Source: CAD feature listing. Evaluate the final solid. Frame: model axes, mm. A direction names the side the tool comes from. Give positions to 0.01 mm unless a question says otherwise; leave off trailing zeros. Loops run counter-clockwise (first coordinate to the right, second up) from the corner with the lowest first, then second, coordinate; pieces in that order, holes last. Notation, with made-up numbers: M 24.25,-31 L 44.25,-31 A27 ccw 44.25,-2 Z; hole C 18.5,-23 d2. An arc over 180 degrees is marked long. Answer in a Markdown table with one row per item.
```python
from build123d import *

# Parameters (mm, degrees)
BOSS_EXTRUDE1_DEPTH         = 2
SKETCH5_R                   = 4.5
SKETCH5_R_2                 = 2.5
BOSS_EXTRUDE2_DEPTH         = 3
SKETCH8_R                   = 1.5
CUT_EXTRUDE2_DEPTH          = 28.531284582
CUT_EXTRUDE3_REACH          = 29.531
SKETCH10_R                  = 0.75
LPATTERN1_COUNT             = 4
LPATTERN1_PITCH             = 3
CIRPATTERN1_COUNT           = 4
CIRPATTERN1_COPY_1_REACH    = 29.531
CIRPATTERN1_COPY_1_SKETCH_R = 0.75
CIRPATTERN1_COPY_2_REACH    = 29.531
CIRPATTERN1_COPY_2_SKETCH_R = 0.75
CIRPATTERN1_COPY_3_REACH    = 29.531
CIRPATTERN1_COPY_3_SKETCH_R = 0.75
CIRPATTERN1_COPY_4_REACH    = 29.531
CIRPATTERN1_COPY_4_SKETCH_R = 0.75
CIRPATTERN1_COPY_5_REACH    = 29.531
CIRPATTERN1_COPY_5_SKETCH_R = 0.75
CIRPATTERN1_COPY_6_REACH    = 29.531
CIRPATTERN1_COPY_6_SKETCH_R = 0.75
CIRPATTERN1_COPY_7_REACH    = 29.531
CIRPATTERN1_COPY_7_SKETCH_R = 0.75
CIRPATTERN1_COPY_8_REACH    = 29.531
CIRPATTERN1_COPY_8_SKETCH_R = 0.75
CIRPATTERN1_COPY_9_REACH    = 29.531
CIRPATTERN1_COPY_9_SKETCH_R = 0.75
SKETCH9_R                   = 4.5
SKETCH9_R_2                 = 3.3
SKETCH9_R_3                 = 2.8
SKETCH9_R_4                 = 1.5
CUT_EXTRUDE4_DEPTH          = 1


with BuildPart() as part:
    # Sketch1 → Boss-Extrude1 (new body)
    with BuildSketch(Plane(origin=(0, 0, 0), x_dir=(1, 0, 0), z_dir=(0, 1, 0))):
        with BuildLine():
            Line((10.343686836, 2.276584719), (4.865650492, -6.089484718))
            ThreePointArc((4.865650492, -6.089484718), (3.897502175, -8.118293207), (4.865650492, -10.147101696))
            Line((4.865650492, -10.147101696), (10.343686836, -18.513171133))
            ThreePointArc((10.343686836, -18.513171133), (10.084686511, -21.022991964), (7.57486568, -21.281992289))
            Line((7.57486568, -21.281992289), (-0.791203757, -15.803955945))
            ThreePointArc((-0.791203757, -15.803955945), (-2.820012246, -14.835807628), (-4.848820735, -15.803955945))
            Line((-4.848820735, -15.803955945), (-13.214890172, -21.281992289))
            ThreePointArc((-13.214890172, -21.281992289), (-15.724711003, -21.022991964), (-15.983711328, -18.513171133))
            Line((-15.983711328, -18.513171133), (-10.505674984, -10.147101696))
            ThreePointArc((-10.505674984, -10.147101696), (-9.537526667, -8.118293207), (-10.505674984, -6.089484718))
            Line((-10.505674984, -6.089484718), (-15.983711328, 2.276584719))
            ThreePointArc((-15.983711328, 2.276584719), (-15.724711003, 4.78640555), (-13.214890172, 5.045405875))
            Line((-13.214890172, 5.045405875), (-4.848820735, -0.432630469))
            ThreePointArc((-4.848820735, -0.432630469), (-2.820012246, -1.400778786), (-0.791203757, -0.432630469))
            Line((-0.791203757, -0.432630469), (7.57486568, 5.045405875))
            ThreePointArc((7.57486568, 5.045405875), (10.084686511, 4.78640555), (10.343686836, 2.276584719))
        make_face()
    extrude(amount=BOSS_EXTRUDE1_DEPTH)

    # Sketch5 → Boss-Extrude2 (add)
    with BuildSketch(Plane(origin=(0, 2, 0), x_dir=(1, 0, 0), z_dir=(0, 1, 0))):
        with Locations(Location((-2.820012246, -8.118293207, 0), (0, 0, 90))):
            Circle(SKETCH5_R)
        with Locations(Location((-2.820012246, -8.118293207, 0), (0, 0, 270))):
            Circle(SKETCH5_R_2, mode=Mode.SUBTRACT)
    extrude(amount=BOSS_EXTRUDE2_DEPTH)

    # Sketch8 → Cut-Extrude2 (cut, through all)
    with BuildSketch(Plane.XZ):
        with Locations(Location((-2.820012246, 8.118293207, 0), (0, 0, 270))):
            Circle(SKETCH8_R)
    extrude(amount=-CUT_EXTRUDE2_DEPTH, mode=Mode.SUBTRACT)

    # Sketch10 → Cut-Extrude3 (cut, up to next)
    with BuildSketch(Plane.XZ, mode=Mode.PRIVATE) as cut_extrude3_sk1:
        with Locations(Location((8.670472948, -3.372191987, 0), (0, 0, 270))):
            Circle(SKETCH10_R)
    cut_extrude3_tool1 = extrude(cut_extrude3_sk1.sketch, amount=-CUT_EXTRUDE3_REACH, mode=Mode.PRIVATE) & part.part
    cut_extrude3 = cut_extrude3_tool1.solids().sort_by_distance((8.670473, 0, -3.372192))[0]
    add(cut_extrude3, mode=Mode.SUBTRACT)

    # LPattern1: Cut-Extrude3 ×4
    with Locations(*[Vector(-0.7071067811865462, 0, 0.7071067811865489) * (i * LPATTERN1_PITCH) for i in range(1, LPATTERN1_COUNT)]):
        add(cut_extrude3, mode=Mode.SUBTRACT)

    # CirPattern1: Cut-Extrude3 ×4 about axis
    cirpattern1_axis = Axis((-2.820012246, 0, 8.118293207), (0, 1, 0))
    for i in range(1, CIRPATTERN1_COUNT):
        add(cut_extrude3.rotate(cirpattern1_axis, i * 360 / CIRPATTERN1_COUNT), mode=Mode.SUBTRACT)

    # CirPattern1 copy 1 sketch → CirPattern1 copy 1 (cut, up to next)
    with BuildSketch(Plane(origin=(-8.81698511, 0, 7.419601305), x_dir=(0, 0, -1), z_dir=(0, -1, 0)), mode=Mode.PRIVATE) as cirpattern1_copy_1_sk1:
        with Locations(Location((8.670472948, -3.372191987, 0), (0, 0, 270))):
            Circle(CIRPATTERN1_COPY_1_SKETCH_R)
    cirpattern1_copy_1_tool1 = extrude(cirpattern1_copy_1_sk1.sketch, amount=-CIRPATTERN1_COPY_1_REACH, mode=Mode.PRIVATE) & part.part
    add(cirpattern1_copy_1_tool1.solids().sort_by_distance((-12.18917711, 0, -1.250871695))[0], mode=Mode.SUBTRACT)

    # CirPattern1 copy 2 sketch → CirPattern1 copy 2 (cut, up to next)
    with BuildSketch(Plane(origin=(-3.518704148, 0, 14.115266071), x_dir=(-1, 0, 0), z_dir=(0, -1, 0)), mode=Mode.PRIVATE) as cirpattern1_copy_2_sk1:
        with Locations(Location((8.670472948, -3.372191987, 0), (0, 0, 270))):
            Circle(CIRPATTERN1_COPY_2_SKETCH_R)
    cirpattern1_copy_2_tool1 = extrude(cirpattern1_copy_2_sk1.sketch, amount=-CIRPATTERN1_COPY_2_REACH, mode=Mode.PRIVATE) & part.part
    add(cirpattern1_copy_2_tool1.solids().sort_by_distance((-12.189177148, 0, 17.487458071))[0], mode=Mode.SUBTRACT)

    # CirPattern1 copy 3 sketch → CirPattern1 copy 3 (cut, up to next)
    with BuildSketch(Plane(origin=(3.176960618, 0, 8.81698511), x_dir=(0, 0, 1), z_dir=(0, -1, 0)), mode=Mode.PRIVATE) as cirpattern1_copy_3_sk1:
        with Locations(Location((8.670472948, -3.372191987, 0), (0, 0, 270))):
            Circle(CIRPATTERN1_COPY_3_SKETCH_R)
    cirpattern1_copy_3_tool1 = extrude(cirpattern1_copy_3_sk1.sketch, amount=-CIRPATTERN1_COPY_3_REACH, mode=Mode.PRIVATE) & part.part
    add(cirpattern1_copy_3_tool1.solids().sort_by_distance((6.549152618, 0, 17.48745811))[0], mode=Mode.SUBTRACT)

    # CirPattern1 copy 4 sketch → CirPattern1 copy 4 (cut, up to next)
    with BuildSketch(Plane(origin=(-6.695664766, 0, 9.540921648), x_dir=(0, 0, -1), z_dir=(0, -1, 0)), mode=Mode.PRIVATE) as cirpattern1_copy_4_sk1:
        with Locations(Location((8.670472948, -3.372191987, 0), (0, 0, 270))):
            Circle(CIRPATTERN1_COPY_4_SKETCH_R)
    cirpattern1_copy_4_tool1 = extrude(cirpattern1_copy_4_sk1.sketch, amount=-CIRPATTERN1_COPY_4_REACH, mode=Mode.PRIVATE) & part.part
    add(cirpattern1_copy_4_tool1.solids().sort_by_distance((-10.067856766, 0, 0.870448648))[0], mode=Mode.SUBTRACT)

    # CirPattern1 copy 5 sketch → CirPattern1 copy 5 (cut, up to next)
    with BuildSketch(Plane(origin=(-1.397383805, 0, 11.993945727), x_dir=(-1, 0, 0), z_dir=(0, -1, 0)), mode=Mode.PRIVATE) as cirpattern1_copy_5_sk1:
        with Locations(Location((8.670472948, -3.372191987, 0), (0, 0, 270))):
            Circle(CIRPATTERN1_COPY_5_SKETCH_R)
    cirpattern1_copy_5_tool1 = extrude(cirpattern1_copy_5_sk1.sketch, amount=-CIRPATTERN1_COPY_5_REACH, mode=Mode.PRIVATE) & part.part
    add(cirpattern1_copy_5_tool1.solids().sort_by_distance((-10.067856805, 0, 15.366137727))[0], mode=Mode.SUBTRACT)

    # CirPattern1 copy 6 sketch → CirPattern1 copy 6 (cut, up to next)
    with BuildSketch(Plane(origin=(1.055640274, 0, 6.695664766), x_dir=(0, 0, 1), z_dir=(0, -1, 0)), mode=Mode.PRIVATE) as cirpattern1_copy_6_sk1:
        with Locations(Location((8.670472948, -3.372191987, 0), (0, 0, 270))):
            Circle(CIRPATTERN1_COPY_6_SKETCH_R)
    cirpattern1_copy_6_tool1 = extrude(cirpattern1_copy_6_sk1.sketch, amount=-CIRPATTERN1_COPY_6_REACH, mode=Mode.PRIVATE) & part.part
    add(cirpattern1_copy_6_tool1.solids().sort_by_distance((4.427832274, 0, 15.366137766))[0], mode=Mode.SUBTRACT)

    # CirPattern1 copy 7 sketch → CirPattern1 copy 7 (cut, up to next)
    with BuildSketch(Plane(origin=(-4.574344422, 0, 11.662241992), x_dir=(0, 0, -1), z_dir=(0, -1, 0)), mode=Mode.PRIVATE) as cirpattern1_copy_7_sk1:
        with Locations(Location((8.670472948, -3.372191987, 0), (0, 0, 270))):
            Circle(CIRPATTERN1_COPY_7_SKETCH_R)
    cirpattern1_copy_7_tool1 = extrude(cirpattern1_copy_7_sk1.sketch, amount=-CIRPATTERN1_COPY_7_REACH, mode=Mode.PRIVATE) & part.part
    add(cirpattern1_copy_7_tool1.solids().sort_by_distance((-7.946536422, 0, 2.991768992))[0], mode=Mode.SUBTRACT)

    # CirPattern1 copy 8 sketch → CirPattern1 copy 8 (cut, up to next)
    with BuildSketch(Plane(origin=(0.723936539, 0, 9.872625384), x_dir=(-1, 0, 0), z_dir=(0, -1, 0)), mode=Mode.PRIVATE) as cirpattern1_copy_8_sk1:
        with Locations(Location((8.670472948, -3.372191987, 0), (0, 0, 270))):
            Circle(CIRPATTERN1_COPY_8_SKETCH_R)
    cirpattern1_copy_8_tool1 = extrude(cirpattern1_copy_8_sk1.sketch, amount=-CIRPATTERN1_COPY_8_REACH, mode=Mode.PRIVATE) & part.part
    add(cirpattern1_copy_8_tool1.solids().sort_by_distance((-7.946536461, 0, 13.244817384))[0], mode=Mode.SUBTRACT)

    # CirPattern1 copy 9 sketch → CirPattern1 copy 9 (cut, up to next)
    with BuildSketch(Plane(origin=(-1.06568007, 0, 4.574344422), x_dir=(0, 0, 1), z_dir=(0, -1, 0)), mode=Mode.PRIVATE) as cirpattern1_copy_9_sk1:
        with Locations(Location((8.670472948, -3.372191987, 0), (0, 0, 270))):
            Circle(CIRPATTERN1_COPY_9_SKETCH_R)
    cirpattern1_copy_9_tool1 = extrude(cirpattern1_copy_9_sk1.sketch, amount=-CIRPATTERN1_COPY_9_REACH, mode=Mode.PRIVATE) & part.part
    add(cirpattern1_copy_9_tool1.solids().sort_by_distance((2.30651193, 0, 13.244817422))[0], mode=Mode.SUBTRACT)

    # Sketch9 → Cut-Extrude4 (cut)
    # profile 1 of 2: a face of its own
    with BuildSketch(Plane.XZ):
        with Locations(Location((-2.820012246, 8.118293207, 0), (0, 0, 270))):
            Circle(SKETCH9_R)
        with Locations(Location((-2.820012246, 8.118293207, 0), (0, 0, 270))):
            Circle(SKETCH9_R_2, mode=Mode.SUBTRACT)
    # profile 2 of 2: a face of its own
    with BuildSketch(Plane.XZ):
        with Locations(Location((-2.820012246, 8.118293207, 0), (0, 0, 270))):
            Circle(SKETCH9_R_3)
        with Locations(Location((-2.820012246, 8.118293207, 0), (0, 0, 270))):
            Circle(SKETCH9_R_4, mode=Mode.SUBTRACT)
    extrude(amount=-CUT_EXTRUDE4_DEPTH, mode=Mode.SUBTRACT)


solid = part.part
```
Q1. Section query A-A (y = 1.4). Give the number of separate pieces and of enclosed holes in the cut face, plus the area to 3 significant figures.
Values follow:
| item | result |
|---|---|
| separate pieces | 1 |
| enclosed holes | 17 |
| area | 378 mm^2 |
Q2. Ray query, probe 1 along X at (y, z) = (1.7, 0.5); probe 2 along Z at (x, y) = (-14.5, 0.2); probe 3 along X at (y, z) = (0.5, -0.75). Return the intervals inside material, ascending. Write a range as from..to.
Values follow:
| item | result |
|---|---|
| probe 1 | -14.17..-10.72, -9.42..-4.79, -0.85..3.78, 5.08..8.53 |
| probe 2 | -5.36..-4.1, -2.65..-0.01, 16.25..18.88, 20.33..21.6 |
| probe 3 | -14.98..-12.75, -11.63..-6.65, 1.01..5.99, 7.11..9.34 |
Q3. Reachability of faces 4 (the cylindrical face through (10.06, 0.99, -4.81)), 5 (the cylindrical face through (-2.622, 0.493, 12.614)), 6 (the flat face through (3.333, 0.986, -2.268)), 7 (the flat face through (7.566, 0.986, 14.272)), 8 (the flat face through (-13.206, 0.986, 1.965)) from +Z, -Z, +X, -X, +Y, -Y: full face, straight path, thin tool, end or side. Return the list, or none.
Values follow:
| item | result |
|---|---|
| face 4 | +Y, -Y |
| face 5 | -Y |
| face 6 | -Z, +Y, -Y |
| face 7 | +X, +Y, -Y |
| face 8 | -X, +Y, -Y |
Q4. Section query C-C (y = 3.2). Output: boundary loops of the cut face in (x, z), plus the area to 3 significant figures.
Values follow:
| item | result |
|---|---|
| outline | C -2.82,8.12 d9; hole C -2.82,8.12 d5 |
| area | 44.0 mm^2 |
Q5. Contact query for flat-ended pins moving along their axis: pin 1 Ø1 at (y, z) = (4, 3.5) entering from +X; pin 2 Ø0.9 at (x, z) = (4.43, 0.87) entering from +Y; pin 3 Ø5.5 at (x, z) = (-2.82, 8.12) entering from -Y; pin 4 Ø2 at (y, z) = (1, 6) entering from -X. Output: stop coordinate, or through.
Values follow:
| item | result |
|---|---|
| pin 1 | x = -1.01 |
| pin 2 | through |
| pin 3 | y = 1 |
| pin 4 | x = -11.22 |
Q6. Section query B-B (z = 11.75). Output: boundary loops of the cut face in (x, y).
Values follow:
| item | result |
|---|---|
| outline | M -11.56,0 L -5.48,0 L -5.48,1 L -0.16,1 L -0.16,0 L 5.92,0 L 5.92,2 L -0.16,2 L -0.16,5 L -5.48,5 L -5.48,2 L -11.56,2 Z |
Q7. Mould query, pull axis Z, two halves, no side actions, for faces 1 (the flat face through (-8.973, 0.986, 18.505)), 2 (the flat face through (-13.283, 0.986, 14.389)), 3 (the cylindrical face through (-2.9, 1, 1.4)). Classes: +Z half, -Z half, draft (parallel to the pull), parting line (faces both ways), or undercut.
Values follow:
| item | result |
|---|---|
| face 1 | +Z half |
| face 2 | undercut |
| face 3 | -Z half |
